```python
from build123d import *

# Parameters (mm, degrees)
SKETCH_1_R      = 3.4
SKETCH_1_R_2    = 3.15
EXTRUDE_1_DEPTH = 175


with BuildPart() as part:
    # Sketch 1 → Extrude 1 (new, symmetric)
    with BuildSketch(Plane.XY):
        with BuildLine():
            Line((-15, 20), (-5.727351849, 20))
            Line((-5.727351849, 20), (-5.727351849, 18.530416438))
            Line((-5.727351849, 18.530416438), (-4.25, 18.530416438))
            Line((-4.25, 18.530416438), (-4.25, 15.732027397))
            Line((-4.25, 15.732027397), (-7.111831817, 15.732027397))
            Line((-7.111831817, 15.732027397), (-7.111831817, 17.7))
            Line((-7.111831817, 17.7), (-10.5, 17.7))
            Line((-10.5, 17.7), (-10.5, 12.479898987))
            Line((-10.5, 12.479898987), (-5.420101013, 7.4))
            Line((-5.420101013, 7.4), (5.420101013, 7.4))
            Line((5.420101013, 7.4), (10.5, 12.479898987))
            Line((10.5, 12.479898987), (10.5, 17.7))
            Line((10.5, 17.7), (7.111831817, 17.7))
            Line((7.111831817, 17.7), (7.111831817, 15.732027397))
            Line((7.111831817, 15.732027397), (4.25, 15.732027397))
            Line((4.25, 15.732027397), (4.25, 18.530416438))
            Line((4.25, 18.530416438), (5.727351849, 18.530416438))
            Line((5.727351849, 18.530416438), (5.727351849, 20))
            Line((5.727351849, 20), (15, 20))
            ThreePointArc((15, 20), (18.535533906, 18.535533906), (20, 15))
            Line((20, 15), (20, 5.727351849))
            Line((20, 5.727351849), (18.530416438, 5.727351849))
            Line((18.530416438, 5.727351849), (18.530416438, 4.25))
            Line((18.530416438, 4.25), (15.732027397, 4.25))
            Line((15.732027397, 4.25), (15.732027397, 7.111831817))
            Line((15.732027397, 7.111831817), (17.7, 7.111831817))
            Line((17.7, 7.111831817), (17.7, 10.5))
            Line((17.7, 10.5), (12.479898987, 10.5))
            Line((12.479898987, 10.5), (7.4, 5.420101013))
            Line((7.4, 5.420101013), (7.4, -5.420101013))
            Line((7.4, -5.420101013), (12.479898987, -10.5))
            Line((12.479898987, -10.5), (17.7, -10.5))
            Line((17.7, -10.5), (17.7, -7.111831817))
            Line((17.7, -7.111831817), (15.732027397, -7.111831817))
            Line((15.732027397, -7.111831817), (15.732027397, -4.25))
            Line((15.732027397, -4.25), (18.530416438, -4.25))
            Line((18.530416438, -4.25), (18.530416438, -5.727351849))
            Line((18.530416438, -5.727351849), (20, -5.727351849))
            Line((20, -5.727351849), (20, -15))
            ThreePointArc((20, -15), (18.535533906, -18.535533906), (15, -20))
            Line((15, -20), (5.727351849, -20))
            Line((5.727351849, -20), (5.727351849, -18.530416438))
            Line((5.727351849, -18.530416438), (4.25, -18.530416438))
            Line((4.25, -18.530416438), (4.25, -15.732027397))
            Line((4.25, -15.732027397), (7.111831817, -15.732027397))
            Line((7.111831817, -15.732027397), (7.111831817, -17.7))
            Line((7.111831817, -17.7), (10.5, -17.7))
            Line((10.5, -17.7), (10.5, -12.479898987))
            Line((10.5, -12.479898987), (5.420101013, -7.4))
            Line((5.420101013, -7.4), (-5.420101013, -7.4))
            Line((-5.420101013, -7.4), (-10.5, -12.479898987))
            Line((-10.5, -12.479898987), (-10.5, -17.7))
            Line((-10.5, -17.7), (-7.111831817, -17.7))
            Line((-7.111831817, -17.7), (-7.111831817, -15.732027397))
            Line((-7.111831817, -15.732027397), (-4.25, -15.732027397))
            Line((-4.25, -15.732027397), (-4.25, -18.530416438))
            Line((-4.25, -18.530416438), (-5.727351849, -18.530416438))
            Line((-5.727351849, -18.530416438), (-5.727351849, -20))
            Line((-5.727351849, -20), (-15, -20))
            ThreePointArc((-15, -20), (-18.535533906, -18.535533906), (-20, -15))
            Line((-20, -15), (-20, -5.727351849))
            Line((-20, -5.727351849), (-18.530416438, -5.727351849))
            Line((-18.530416438, -5.727351849), (-18.530416438, -4.25))
            Line((-18.530416438, -4.25), (-15.732027397, -4.25))
            Line((-15.732027397, -4.25), (-15.732027397, -7.111831817))
            Line((-15.732027397, -7.111831817), (-17.7, -7.111831817))
            Line((-17.7, -7.111831817), (-17.7, -10.5))
            Line((-17.7, -10.5), (-12.479898987, -10.5))
            Line((-12.479898987, -10.5), (-7.4, -5.420101013))
            Line((-7.4, -5.420101013), (-7.4, 5.420101013))
            Line((-7.4, 5.420101013), (-12.479898987, 10.5))
            Line((-12.479898987, 10.5), (-17.7, 10.5))
            Line((-17.7, 10.5), (-17.7, 7.111831817))
            Line((-17.7, 7.111831817), (-15.732027397, 7.111831817))
            Line((-15.732027397, 7.111831817), (-15.732027397, 4.25))
            Line((-15.732027397, 4.25), (-18.530416438, 4.25))
            Line((-18.530416438, 4.25), (-18.530416438, 5.727351849))
            Line((-18.530416438, 5.727351849), (-20, 5.727351849))
            Line((-20, 5.727351849), (-20, 15))
            ThreePointArc((-20, 15), (-18.535533906, 18.535533906), (-15, 20))
        make_face()
        Circle(SKETCH_1_R, mode=Mode.SUBTRACT)
        with Locations((-15, 15)):
            Circle(SKETCH_1_R_2, mode=Mode.SUBTRACT)
        with Locations(Location((15, 15, 0), (0, 0, 180))):
            Circle(SKETCH_1_R_2, mode=Mode.SUBTRACT)
        with Locations((15, -15)):
            Circle(SKETCH_1_R_2, mode=Mode.SUBTRACT)
        with Locations(Location((-15, -15, 0), (0, 0, 180))):
            Circle(SKETCH_1_R_2, mode=Mode.SUBTRACT)
    extrude(amount=EXTRUDE_1_DEPTH, both=True)


solid = part.part
```
Can you work these out from the model? Positions are in its coordinate system, mm. A direction names the side the tool comes from. Round coordinates to 2 decimals unless told otherwise and drop trailing zeros. Loops run counter-clockwise (first coordinate to the right, second up) from the corner with the lowest first, then second, coordinate; pieces in that order, holes last. Notation, with made-up numbers: (30, -12.5) -> (85, -12.5) arc R12 ccw to (85, -0.5) -> close; hole circle Ø2 at (28.5, 9.5). An arc over 180 degrees is marked (long way). Answer in a Markdown table with one row per item.
Item 1: On a 3-axis mill with a long thin cutter (end or side, diameter ignored), from which of +Z, -Z, +X, -X, +Y, -Y can I reach the whole of each face in a straight line? I mean faces 1 (the flat face through (-7.4, 0, 2)), 2 (the flat face through (-20, 10, 2)). Say none if no direction works.
Answer block:
| item | result |
|---|---|
| face 1 | +Z, -Z |
| face 2 | +Z, -Z, -X, +Y, -Y |
Item 2: Will these pins go through, and if not, where does the flat tip stop? P1, Ø1.2, axis at y = 5, z = 15.5, coming from the -X side; P2, Ø5.5, axis at x = 15, y = 15, coming from the +Z side; P3, Ø5.5, axis at y = -2, z = -64, coming from the +X side; P4, Ø1.2, axis at x = -19, z = -3, coming from the -Y side.
Answer block:
| item | result |
|---|---|
| P1 | x = -18.53 |
| P2 | through |
| P3 | x = 18.53 |
| P4 | y = -18.67 |
Item 3: We'd pull the mould along Y, two halves only. Please class faces 3 (the flat face through (-10, 20, 2)), 4 (the cylindrical face through (-0.74, -3.32, -2.45)), 5 (the flat face through (-20, -10, 2)): released by +Y, released by -Y, zero draft, split by the parting line, or undercut.
Answer block:
| item | result |
|---|---|
| face 3 | released by +Y |
| face 4 | undercut |
| face 5 | zero draft |
Item 4: Suppose I cut it at C-C, the plane z = 130.5. Give the number of separate pieces and of enclosed holes in the cut face, plus the area to 3 significant figures.
Answer block:
| item | result |
|---|---|
| separate pieces | 1 |
| enclosed holes | 5 |
| area | 605 mm² |
Item 5: If I drill on probe 1 along Y at (x, z) = (15, 37); probe 2 along Y at (x, z) = (0, -94); probe 3 along Y at (x, z) = (-16, 79), over which ranges is the centre line in solid material (lowest first)?
Answer block:
| item | result |
|---|---|
| probe 1 | -20 to -18.15, -11.85 to -10.5, 10.5 to 11.85, 18.15 to 20 |
| probe 2 | -7.4 to -3.4, 3.4 to 7.4 |
| probe 3 | -19.9 to -17.99, -12.01 to -10.5, -7.11 to -4.25, 4.25 to 7.11, 10.5 to 12.01, 17.99 to 19.9 |
Item 6: Suppose I cut it at A-A, the plane x = 0. List the corners of the cut face in (y, z) for me.
Answer block:
| item | result |
|---|---|
| outline | (-7.4, -175) -> (-3.4, -175) -> (-3.4, 175) -> (-7.4, 175) -> close; (3.4, -175) -> (7.4, -175) -> (7.4, 175) -> (3.4, 175) -> close |
